```python
from build123d import *

# Parameters (mm, degrees)
SKETCH1_R           = 5
BOSS_EXTRUDE1_DEPTH = 6.5
SKETCH2_R           = 5
SKETCH2_R_2         = 2.5
CUT_EXTRUDE1_DEPTH  = 9
CUT_EXTRUDE2_DEPTH  = 4


with BuildPart() as part:
    # Sketch1 → Boss-Extrude1 (new body, symmetric)
    with BuildSketch(Plane(origin=(0, 0, 0), x_dir=(1, 0, 0), z_dir=(0, 1, 0))):
        Circle(SKETCH1_R)
    extrude(amount=BOSS_EXTRUDE1_DEPTH, both=True)

    # Sketch2 → Cut-Extrude1 (cut)
    with BuildSketch(Plane.XZ.offset(6.5)):
        Circle(SKETCH2_R)
        Circle(SKETCH2_R_2, mode=Mode.SUBTRACT)
    extrude(amount=-CUT_EXTRUDE1_DEPTH, mode=Mode.SUBTRACT)

    # Sketch4 → Cut-Extrude2 (cut)
    with BuildSketch(Plane(origin=(0, 6.5, 0), x_dir=(1, 0, 0), z_dir=(0, 1, 0))):
        with BuildLine():
            Line((-4.999938781, -0.024742442), (-2.521396974, 4.317702781))
            ThreePointArc((-2.521396974, 4.317702781), (-4.342445223, 2.478541807), (-4.999938781, -0.024742442))
        make_face()
        with BuildLine():
            Line((-2.478541807, -4.342445223), (-4.999938781, -0.024742442))
            ThreePointArc((-4.999938781, -0.024742442), (-4.317702781, -2.521396974), (-2.478541807, -4.342445223))
        make_face()
        with BuildLine():
            ThreePointArc((-2.478541807, -4.342445223), (0.024742442, -4.999938781), (2.521396974, -4.317702781))
            Line((2.521396974, -4.317702781), (-2.478541807, -4.342445223))
        make_face()
        with BuildLine():
            ThreePointArc((5, 0), (4.999984695, 0.012371259), (4.999938781, 0.024742442))
            Line((4.999938781, 0.024742442), (2.521396974, -4.317702781))
            ThreePointArc((2.521396974, -4.317702781), (4.336299394, -2.489278523), (5, 0))
        make_face()
        with BuildLine():
            ThreePointArc((4.999938781, 0.024742442), (4.317702781, 2.521396974), (2.478541807, 4.342445223))
            Line((2.478541807, 4.342445223), (4.999938781, 0.024742442))
        make_face()
        with BuildLine():
            Line((-2.521396974, 4.317702781), (2.478541807, 4.342445223))
            ThreePointArc((2.478541807, 4.342445223), (-0.024742442, 4.999938781), (-2.521396974, 4.317702781))
        make_face()
    extrude(amount=-CUT_EXTRUDE2_DEPTH, mode=Mode.SUBTRACT)

    # Sketch5 → Cut-Revolve1 (revolve, cut)
    with BuildSketch(Plane.XY):
        with BuildLine():
            Line((-3.722260503, 6.5), (-3.722260503, 8.060451161))
            Line((-3.722260503, 8.060451161), (-6.740732256, 6.10732238))
            Line((-6.740732256, 6.10732238), (-4.999938781, 5.059459129))
            Line((-4.999938781, 5.059459129), (-4.999938781, 5.5))
            ThreePointArc((-4.999938781, 5.5), (-4.707045562, 6.207106781), (-3.999938781, 6.5))
            Line((-3.999938781, 6.5), (-3.722260503, 6.5))
        make_face()
    revolve(axis=Axis((0, 0, 0), (0, 1, 0)), mode=Mode.SUBTRACT)


solid = part.part
```
CAD build for the part. Positions are in the model's coordinates, mm. A direction names the side the tool comes from. Round coordinates to 2 decimals unless told otherwise and drop trailing zeros. Order: outer loops, then holes, each group sorted by start corner. A loop starts at its lowest first (then second) coordinate and runs counter-clockwise, first axis right, second up.
Item 1: Pin check, flat tips, straight feed: pin 1 (4 mm diameter, centred on x = -4, y = 3, fed in from -Z); pin 2 (2 mm diameter, centred on x = 2, y = 1, fed in from +Z). Stop position of each tip, or through.
Item 2: Tool access for faces 1 (the face through (-0.54, -2.06, -2.44)), 2 (the face through (3.722, 4.5, -2.214)): list every direction of +Z, -Z, +X, -X, +Y, -Y with a clear straight run to the whole face (end or side of a thin tool).
Item 3: Saw through at C-C on y = -3.25. Write the cut outline in (x, z).
Item 4: Probe line 1 along Y through (x, z) = (1.25, 3); line 2 along X through (y, z) = (-4.5, -0.25); line 3 along Y through (x, z) = (3, 3.25). List the from-to ranges inside material, lowest first.
Item 5: Saw through at A-A on y = 3.75. Write the cut outline in (x, z).
Item 6: Saw through at B-B on x = 0. Write the cut outline in (y, z), then the cut area to 3 significant figures.
Reported:
1. pin 1: stops at z = -4.32
1. pin 2: stops at z = 2.29
2. face 1: -Y
2. face 2: -Z, +X, +Y, -Y
3. outline: circle Ø5 at (0, 0)
4. line 1: y = 2.5 to 6.5
4. line 2: x = -2.49 to 2.49
4. line 3: y = 2.5 to 6.41
5. outline: (-5, 0.02) - (-2.52, -4.32) - (2.48, -4.34) - (5, -0.02) - (2.52, 4.32) - (-2.48, 4.34) - close
6. outline: (-6.5, -2.5) - (2.5, -2.5) - (2.5, -4.33) - (6.44, -4.33) arc R1 ccw to (6.5, -4) - (6.5, 4) arc R1 ccw to (6.44, 4.33) - (2.5, 4.33) - (2.5, 2.5) - (-6.5, 2.5) - close
6. area: 79.6 mm2
